Job drawing, mm, ordinate dimensions from the low corner. One solid piece. Coordinates: 2 decimals unless noted, no trailing zeros. Loops run counter-clockwise (first coordinate to the right, second up) from the corner with the lowest first, then second, coordinate; pieces in that order, holes last. Notation, with made-up numbers: (85, 9.25) -> (111, 9.25) arc R18 ccw to (111, 23.25) -> close; hole circle Ø6 at (9.5, 35.25). An arc over 180 degrees is marked (long way). Use one line per item in the form item = value. Start each with the question number.
(1) Drill centre lines: L1, parallel to X at y = 271.5, z = 11.75 (3 decimals); L2, parallel to Z at x = 72.5, y = 49 (3 decimals); L3, parallel to X at y = 178.5, z = 21. Where is each one in solid material? Low to high. Write a range as [from, to].
(2) Pin check, flat tip, straight feed: P1, Ø1, axis at x = 20, y = 96.5, coming from the -Z side (3 decimals). Stop position of the tip, or through.
(3) Band-saw the part on C-C on x = 61.5. Give the cut face in (y, z) (3 decimals).
(4) Mould opens along X. For the marked faces 1, 2 and 3 say: +X half, -X half, draft (parallel to the pull), parting line (faces both ways), or undercut.
(5) Band-saw the part on B-B on y = 277. Give the cut face in (x, z) (3 decimals).
(6) Band-saw the part on A-A on z = 10.75. Give the cut face in (x, y) (3 decimals).
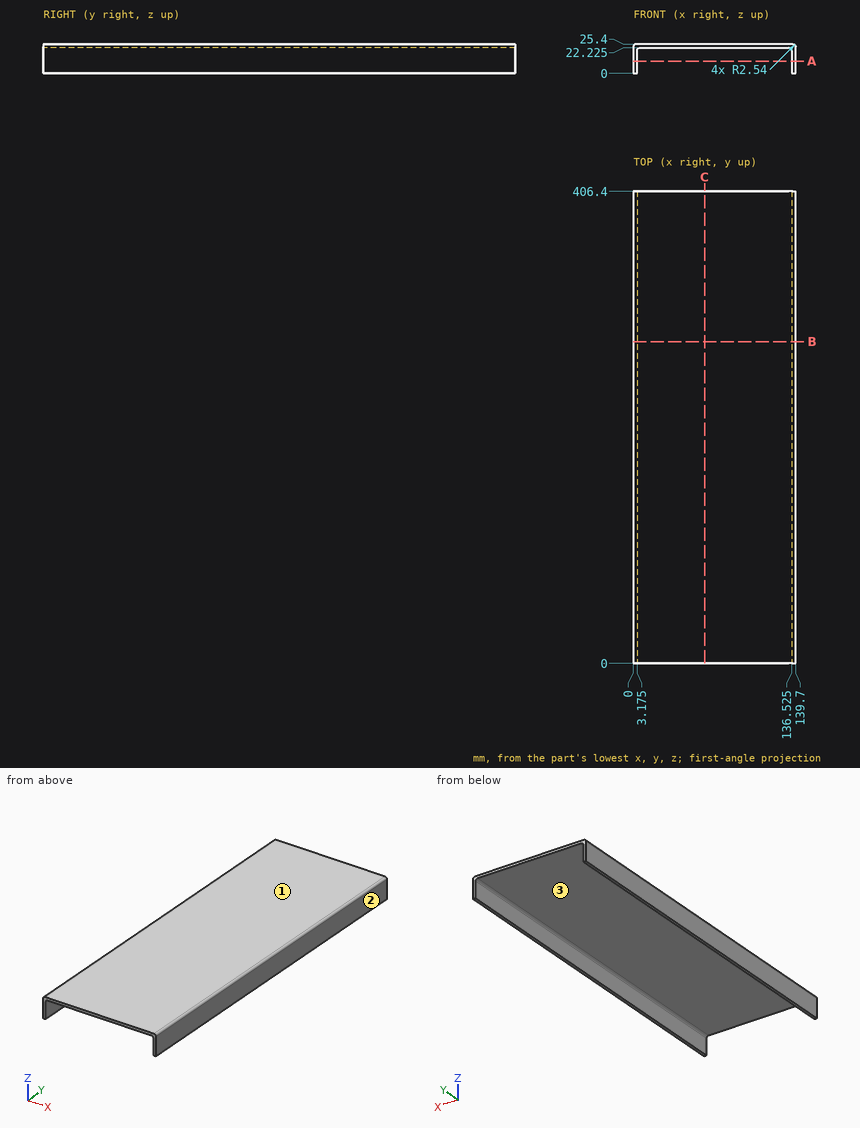
A:
q1.L1 = [0, 3.175], [136.525, 139.7]
q1.L2 = [22.225, 25.4]
q1.L3 = [0, 3.54], [136.16, 139.7]
q2.P1 = 22.225
q3.outline = (0, 22.225) -> (406.4, 22.225) -> (406.4, 25.4) -> (0, 25.4) -> close
q4.face_1 = draft
q4.face_2 = +X half
q4.face_3 = undercut
q5.outline = (0, 0) -> (3.175, 0) -> (3.175, 19.685) arc R2.54 cw to (5.715, 22.225) -> (133.985, 22.225) arc R2.54 cw to (136.525, 19.685) -> (136.525, 0) -> (139.7, 0) -> (139.7, 22.86) arc R2.54 ccw to (137.16, 25.4) -> (2.54, 25.4) arc R2.54 ccw to (0, 22.86) -> close
q6.outline = (0, 0) -> (3.175, 0) -> (3.175, 406.4) -> (0, 406.4) -> close; (136.525, 0) -> (139.7, 0) -> (139.7, 406.4) -> (136.525, 406.4) -> close
